Can you work these out from the model? Positions are in its coordinate system, mm. Coordinates: 2 decimals unless noted, no trailing zeros. Loops run counter-clockwise (first coordinate to the right, second up) from the corner with the lowest first, then second, coordinate; pieces in that order, holes last. Notation, with made-up numbers: (-22.5, 32.25) - (20.5, 32.25) arc R22 cw to (20.5, 58.25) - close; hole circle Ø10 at (56.25, 64.25). An arc over 180 degrees is marked (long way). Put each result on its own line as item: value. Start each with the question number.
from build123d import *

# Parameters (mm, degrees)
CROQUIS1_R              = 1.5
CROQUIS1_R_2            = 1
CROQUIS1_R_3            = 1.004910311
CROQUIS1_R_4            = 2.25
SALIENTE_EXTRUIR1_DEPTH = 4


with BuildPart() as part:
    # Croquis1 → Saliente-Extruir1 (new body)
    with BuildSketch(Plane.XY):
        with BuildLine():
            Line((-72.974134086, -82.873629023), (14, 4.100505063))
            Line((14, 4.100505063), (100.974134086, -82.873629023))
            ThreePointArc((100.974134086, -82.873629023), (110.873629023, -82.873629023), (110.873629023, -72.974134086))
            Line((110.873629023, -72.974134086), (23.899494937, 14))
            Line((23.899494937, 14), (110.873629023, 100.974134086))
            ThreePointArc((110.873629023, 100.974134086), (110.873629023, 110.873629023), (100.974134086, 110.873629023))
            Line((100.974134086, 110.873629023), (14, 23.899494937))
            Line((14, 23.899494937), (-72.974134086, 110.873629023))
            ThreePointArc((-72.974134086, 110.873629023), (-82.873629023, 110.873629023), (-82.873629023, 100.974134086))
            Line((-82.873629023, 100.974134086), (4.100505063, 14))
            Line((4.100505063, 14), (-82.873629023, -72.974134086))
            ThreePointArc((-82.873629023, -72.974134086), (-82.873629023, -82.873629023), (-72.974134086, -82.873629023))
        make_face()
        with Locations((7, 7)):
            Circle(CROQUIS1_R, mode=Mode.SUBTRACT)
        with Locations((21, 7)):
            Circle(CROQUIS1_R, mode=Mode.SUBTRACT)
        with Locations((-73.423881554, -77.923881554)):
            Circle(CROQUIS1_R_2, mode=Mode.SUBTRACT)
        with Locations((-77.923881554, -82.423881554)):
            Circle(CROQUIS1_R_3, mode=Mode.SUBTRACT)
        with Locations((-82.423881554, -77.923881554)):
            Circle(CROQUIS1_R_2, mode=Mode.SUBTRACT)
        with Locations((-77.923881554, -73.423881554)):
            Circle(CROQUIS1_R_2, mode=Mode.SUBTRACT)
        with Locations((7, 21)):
            Circle(CROQUIS1_R, mode=Mode.SUBTRACT)
        with Locations((110.423881554, -77.923881554)):
            Circle(CROQUIS1_R_2, mode=Mode.SUBTRACT)
        with Locations((105.923881554, -82.423881554)):
            Circle(CROQUIS1_R_2, mode=Mode.SUBTRACT)
        with Locations((101.423881554, -77.923881554)):
            Circle(CROQUIS1_R_2, mode=Mode.SUBTRACT)
        with Locations((105.923881554, -73.423881554)):
            Circle(CROQUIS1_R_2, mode=Mode.SUBTRACT)
        with Locations((-73.423881554, 105.923881554)):
            Circle(CROQUIS1_R_2, mode=Mode.SUBTRACT)
        with Locations((-77.923881554, 101.423881554)):
            Circle(CROQUIS1_R_2, mode=Mode.SUBTRACT)
        with Locations((-82.423881554, 105.923881554)):
            Circle(CROQUIS1_R_2, mode=Mode.SUBTRACT)
        with Locations((-77.923881554, 110.423881554)):
            Circle(CROQUIS1_R_2, mode=Mode.SUBTRACT)
        with Locations((21, 21)):
            Circle(CROQUIS1_R, mode=Mode.SUBTRACT)
        with Locations((110.423881554, 105.923881554)):
            Circle(CROQUIS1_R_2, mode=Mode.SUBTRACT)
        with Locations((105.923881554, 101.423881554)):
            Circle(CROQUIS1_R_2, mode=Mode.SUBTRACT)
        with Locations((101.423881554, 105.923881554)):
            Circle(CROQUIS1_R_2, mode=Mode.SUBTRACT)
        with Locations((105.923881554, 110.423881554)):
            Circle(CROQUIS1_R_2, mode=Mode.SUBTRACT)
        with Locations((-77.923881554, -77.923881554)):
            Circle(CROQUIS1_R_4, mode=Mode.SUBTRACT)
        with Locations((105.923881554, -77.923881554)):
            Circle(CROQUIS1_R_4, mode=Mode.SUBTRACT)
        with Locations((105.923881554, 105.923881554)):
            Circle(CROQUIS1_R_4, mode=Mode.SUBTRACT)
        with Locations((-77.923881554, 105.923881554)):
            Circle(CROQUIS1_R_4, mode=Mode.SUBTRACT)
    extrude(amount=SALIENTE_EXTRUIR1_DEPTH)


solid = part.part
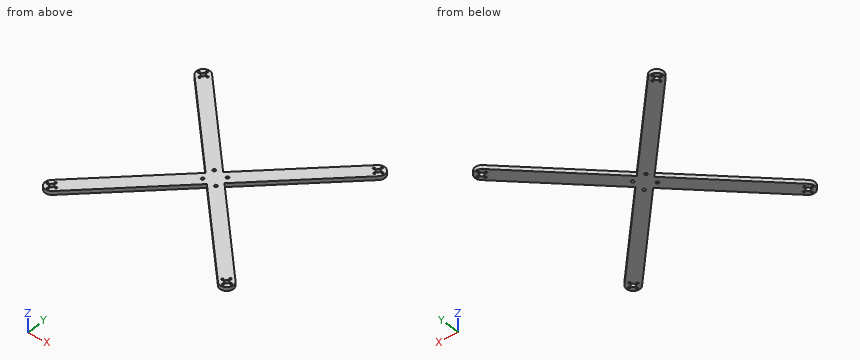
Q1. I want a section at B-B on y = -43. List the corners of the cut face in (x, z) for me, and give its area (3 significant figures).
Q2. Will these pins go through, and if not, where does the flat tip stop? pin 1 (3 mm diameter, centred on x = 105.92, y = 110.42, fed in from +Z); pin 2 (2 mm diameter, centred on y = 61, z = 3, fed in from -X); pin 3 (1 mm diameter, centred on y = 37.5, z = 3, fed in from -X); pin 4 (2 mm diameter, centred on x = 30, z = 0.5, fed in from -Y).
Q3. I want a section at A-A on x = -45. List the corners of the cut face in (y, z) for me.
Q4. Please list where these lines run through material, in increasing order: line 1 along X through (y, z) = (104, 0.65); line 2 along X through (y, z) = (6, 3.1); line 3 along Y through (x, z) = (7, 1.4). Write a range as [from, to].
Q5. I want a section at C-C on z = 3.3. Count the separate pieces of the cut face and the enclosed holes in it, and give its area (3 significant figures).
Calculated:
1. outline: (-52.9, 0) - (-33.1, 0) - (-33.1, 4) - (-52.9, 4) - close; (61.1, 0) - (80.9, 0) - (80.9, 4) - (61.1, 4) - close
1. area: 158 mm2
2. pin 1: z = 4
2. pin 2: x = -43.9
2. pin 3: x = -19.9
2. pin 4: y = -12.9
3. outline: (-54.9, 0) - (-35.1, 0) - (-35.1, 4) - (-54.9, 4) - close; (63.1, 0) - (82.9, 0) - (82.9, 4) - (63.1, 4) - close
4. line 1: [-84.65, -79.09], [-76.76, -66.1], [94.1, 104.76], [107.09, 112.65]
4. line 2: [-3.9, 5.88], [8.12, 19.88], [22.12, 31.9]
4. line 3: [-2.9, 5.5], [8.5, 19.5], [22.5, 30.9]
5. separate pieces: 1
5. enclosed holes: 24
5. area: 7,250 mm2
